Verification items for the finished model (mm, model axes). A direction names the side the tool comes from. Give positions to 0.01 mm unless a question says otherwise; leave off trailing zeros. Use a Markdown table: item, result.
from build123d import *

# Parameters (mm, degrees)
SKETCH1_W                = 94
SKETCH1_H                = 130
BOSS_EXTRUDE1_DEPTH      = 9.5
SKETCH2_W                = 90.5
SKETCH2_H                = 126.5
CUT_EXTRUDE1_DEPTH       = 2.5
SKETCH3_W                = 70
SKETCH3_H                = 24
CUT_EXTRUDE2_DEPTH       = 8
SKETCH4_W                = 70
SKETCH4_H                = 77
CUT_EXTRUDE3_DEPTH       = 2
SKETCH5_W                = 23
SKETCH5_H                = 3.5
CUT_EXTRUDE4_DEPTH       = 8.5
SKETCH6_W                = 6
SKETCH6_H                = 18
CUT_EXTRUDE5_DEPTH       = 3.5
SKETCH7_W                = 43
SKETCH7_H                = 7.5
CUT_EXTRUDE6_DEPTH       = 3
FILLET1_R                = 2
SKETCH9_R                = 2.75
CUT_EXTRUDE7_DEPTH       = 5
SKETCH12_W               = 6.2
SKETCH12_H               = 6.2
CUT_EXTRUDE9_DEPTH       = 3
SKETCH13_W               = 3.2
SKETCH13_H               = 6.2
CUT_EXTRUDE10_DEPTH      = 6
CUT_EXTRUDE10_DEPTH_BACK = 5.5
FILLET2_R                = 1
SKETCH14_R               = 4
BOSS_EXTRUDE2_DEPTH      = 3
SKETCH15_R               = 2.8
CUT_EXTRUDE11_DEPTH      = 1.5
SKETCH16_R               = 2.4
CUT_EXTRUDE12_DEPTH      = 1.5
SKETCH18_W               = 4
SKETCH18_H               = 6
SKETCH18_W_2             = 2
SKETCH18_H_2             = 4
SKETCH18_H_3             = 1
BOSS_EXTRUDE3_DEPTH      = 1


with BuildPart() as part:
    # Sketch1 → Boss-Extrude1 (new body)
    with BuildSketch(Plane(origin=(0, 7, 0), x_dir=(1, 0, 0), z_dir=(0, 1, 0))):
        with Locations((47, 65)):
            Rectangle(SKETCH1_W, SKETCH1_H)
    extrude(amount=-BOSS_EXTRUDE1_DEPTH)

    # Sketch2 → Cut-Extrude1 (cut)
    with BuildSketch(Plane.XZ.offset(2.5)):
        with Locations((47, -65)):
            Rectangle(SKETCH2_W, SKETCH2_H)
    extrude(amount=-CUT_EXTRUDE1_DEPTH, mode=Mode.SUBTRACT)

    # Sketch3 → Cut-Extrude2 (cut, through all)
    with BuildSketch(Plane.XZ):
        with Locations((47, -100)):
            Rectangle(SKETCH3_W, SKETCH3_H)
    extrude(amount=-CUT_EXTRUDE2_DEPTH, mode=Mode.SUBTRACT)

    # Sketch4 → Cut-Extrude3 (cut)
    with BuildSketch(Plane(origin=(0, 7, 0), x_dir=(-1, 0, 0), z_dir=(0, 1, 0))):
        with Locations((-47, -44.5)):
            Rectangle(SKETCH4_W, SKETCH4_H)
    extrude(amount=-CUT_EXTRUDE3_DEPTH, mode=Mode.SUBTRACT)

    # Sketch5 → Cut-Extrude4 (cut, through all)
    with BuildSketch(Plane(origin=(0, 5, 0), x_dir=(-1, 0, 0), z_dir=(0, 1, 0))):
        with Locations((-39, -9.25)):
            Rectangle(SKETCH5_W, SKETCH5_H)
    extrude(amount=-CUT_EXTRUDE4_DEPTH, mode=Mode.SUBTRACT)

    # Sketch6 → Cut-Extrude5 (cut)
    with BuildSketch(Plane.XZ):
        with Locations((85, -100)):
            Rectangle(SKETCH6_W, SKETCH6_H)
    extrude(amount=-CUT_EXTRUDE5_DEPTH, mode=Mode.SUBTRACT)

    # Sketch7 → Cut-Extrude6 (cut)
    with BuildSketch(Plane.XZ):
        with Locations((33.5, -115.75)):
            Rectangle(SKETCH7_W, SKETCH7_H)
    extrude(amount=-CUT_EXTRUDE6_DEPTH, mode=Mode.SUBTRACT)

    # Fillet1
    fillet1_edges = [part.edges().sort_by_distance(p)[0] for p in [
        (94, 7, -65),
        (47, 7, 0),
        (0, 7, -65),
        (47, 7, -130),
        (94, 2.25, -130),
        (94, 2.25, 0),
        (0, 2.25, 0),
        (0, 2.25, -130),
    ]]
    fillet(fillet1_edges, radius=FILLET1_R)

    # Sketch9 → Cut-Extrude7 (cut)
    with BuildSketch(Plane(origin=(0, 5, 0), x_dir=(1, 0, 0), z_dir=(0, 1, 0))):
        with Locations((74, 58)):
            Circle(SKETCH9_R)
    extrude(amount=-CUT_EXTRUDE7_DEPTH, mode=Mode.SUBTRACT)

    # Sketch12 → Cut-Extrude9 (cut)
    with BuildSketch(Plane(origin=(0, 5, 0), x_dir=(1, 0, 0), z_dir=(0, 1, 0))):
        with Locations((74, 31)):
            Rectangle(SKETCH12_W, SKETCH12_H)
    extrude(amount=-CUT_EXTRUDE9_DEPTH, mode=Mode.SUBTRACT)

    # Sketch13 → Cut-Extrude10 (cut, two sides)
    with BuildSketch(Plane(origin=(0, 2, 0), x_dir=(1, 0, 0), z_dir=(0, 1, 0))) as cut_extrude10_sk:
        with Locations((74, 31)):
            Rectangle(SKETCH13_W, SKETCH13_H)
    extrude(amount=CUT_EXTRUDE10_DEPTH, mode=Mode.SUBTRACT)
    extrude(cut_extrude10_sk.sketch, amount=-CUT_EXTRUDE10_DEPTH_BACK, mode=Mode.SUBTRACT)

    # Fillet2
    fillet2_edges = [part.edges().sort_by_distance(p)[0] for p in [
        (77.1, 3.5, -34.1),
        (77.1, 3.5, -27.9),
        (70.9, 3.5, -27.9),
        (70.9, 3.5, -34.1),
    ]]
    fillet(fillet2_edges, radius=FILLET2_R)

    # Sketch14 → Boss-Extrude2 (add)
    with BuildSketch(Plane.XZ):
        with Locations((74, -58)):
            Circle(SKETCH14_R)
    extrude(amount=BOSS_EXTRUDE2_DEPTH)

    # Sketch15 → Cut-Extrude11 (cut)
    with BuildSketch(Plane(origin=(0, 0, 0), x_dir=(1, 0, 0), z_dir=(0, 1, 0))):
        with Locations((74, 58)):
            Circle(SKETCH15_R)
    extrude(amount=-CUT_EXTRUDE11_DEPTH, mode=Mode.SUBTRACT)

    # Sketch16 → Cut-Extrude12 (cut)
    with BuildSketch(Plane(origin=(0, -1.5, 0), x_dir=(1, 0, 0), z_dir=(0, 1, 0))):
        with Locations((74, 58)):
            Circle(SKETCH16_R)
    extrude(amount=-CUT_EXTRUDE12_DEPTH, mode=Mode.SUBTRACT)

    # Sketch18 → Boss-Extrude3 (add)
    with BuildSketch(Plane(origin=(0, 7, 0), x_dir=(1, 0, 0), z_dir=(0, 1, 0))):
        Polygon((17, 122), (17, 118), (19, 118), (19.993343468, 118), (19.993343468, 117), (15.993343468, 117), (15.993343468, 123), (19.993343468, 123), (19.993343468, 122), (19, 122), align=None)
        Polygon((66.993343468, 122), (63.993343468, 122), (63.993343468, 120.5), (66.993343468, 120.5), (66.993343468, 117), (62.993343468, 117), (62.993343468, 118), (65.993343468, 118), (65.993343468, 119.5), (62.993343468, 119.5), (62.993343468, 123), (66.993343468, 123), align=None)
        with Locations((23.493343468, 120)):
            Rectangle(SKETCH18_W, SKETCH18_H)
        with Locations((23.493343468, 120)):
            Rectangle(SKETCH18_W_2, SKETCH18_H_2, mode=Mode.SUBTRACT)
        Polygon((27.993343468, 122), (27.993343468, 118), (29.109404955, 118), (30.993343468, 118), (30.993343468, 117), (26.993343468, 117), (26.993343468, 123), (27.993343468, 123), align=None)
        with Locations((34.493343468, 120)):
            Rectangle(SKETCH18_W, SKETCH18_H)
        with Locations((34.493343468, 120)):
            Rectangle(SKETCH18_W_2, SKETCH18_H_2, mode=Mode.SUBTRACT)
        Polygon((49.493343468, 122), (50.493343468, 122), (50.493343468, 123), (46.493343468, 123), (46.493343468, 119.5), (47.493343468, 119.5), (49.493343468, 119.5), (49.493343468, 118), (47.956084084, 118), (46.493343468, 118), (46.493343468, 117), (50.493343468, 117), (50.493343468, 120.5), (49.493343468, 120.5), (47.493343468, 120.5), (47.493343468, 122), align=None)
        Polygon((37.993343468, 123), (41.993343468, 123), (41.993343468, 120), (40.353343468, 120), (41.993343468, 118.2), (41.993343468, 117), (40.993343468, 117), (40.993343468, 117.812757926), (39.000522912, 120), (38.993343468, 120), (38.993343468, 118.442496016), (38.993343468, 117), (37.993343468, 117), align=None)
        with Locations((39.993343468, 121.5)):
            Rectangle(SKETCH18_W_2, SKETCH18_H_3, mode=Mode.SUBTRACT)
        Polygon((55.993343468, 122), (52.993343468, 122), (52.993343468, 120.5), (55.993343468, 120.5), (55.993343468, 119.5), (52.993343468, 119.5), (52.993343468, 118), (55.993343468, 118), (55.993343468, 117), (51.993343468, 117), (51.993343468, 123), (55.993343468, 123), align=None)
        Polygon((58.493343468, 123), (60.493343468, 119.163331999), (60.493343468, 123), (61.493343468, 123), (61.493343468, 117), (60.493343468, 117), (58.493343468, 120.836668001), (58.493343468, 117), (57.493343468, 117), (57.493343468, 123), align=None)
        with Locations((70.493343468, 120)):
            Rectangle(SKETCH18_W, SKETCH18_H)
        with Locations((70.493343468, 120)):
            Rectangle(SKETCH18_W_2, SKETCH18_H_2, mode=Mode.SUBTRACT)
        Polygon((74.993343468, 117), (74.993343468, 120), (75.000522912, 120), (76.993343468, 117.812757926), (76.993343468, 117), (77.993343468, 117), (77.993343468, 118.2), (76.353343468, 120), (77.993343468, 120), (77.993343468, 123), (73.993343468, 123), (73.993343468, 117), align=None)
        with Locations((75.993343468, 121.5)):
            Rectangle(SKETCH18_W_2, SKETCH18_H_3, mode=Mode.SUBTRACT)
    extrude(amount=BOSS_EXTRUDE3_DEPTH)


solid = part.part
(1) Draft check along Z on faces 1 (the flat face through (47, 5, -44)), 2 (the flat face through (40, 8, -120.7)). Enter one of: +Z half, -Z half, draft (parallel to the pull), parting line (faces both ways), or undercut.
Results below:
| item | result |
|---|---|
| face 1 | undercut |
| face 2 | draft |
(2) Gauge pin test, flat ends, axial feed: P1, Ø6.5, axis at x = 85, z = -101, coming from the -Y side; P2, Ø5, axis at x = 17.5, z = -22, coming from the +Y side; P3, Ø0.5, axis at x = 48.5, y = 7.5, coming from the +Z side. Record the tip position at first contact, or that the pin passes through.
Results below:
| item | result |
|---|---|
| P1 | y = 0 |
| P2 | y = 5 |
| P3 | z = -117 |
(3) Material ranges on line 1 (Z direction, x = 74, y = -1.9); line 2 (Z direction, x = 74, y = 1.05); line 3 (X direction, y = 2.85, z = -58), recorded low to high.
Results below:
| item | result |
|---|---|
| line 1 | -130 to -128.25, -62 to -60.4, -55.6 to -54, -1.75 to 0 |
| line 2 | -130 to -112, -88 to -60.75, -55.25 to -34.1, -27.9 to 0 |
| line 3 | 0 to 71.25, 76.75 to 94 |
(4) Set-up check for faces 3 (the flat face through (0, 1, -64)), 4 (the flat face through (88, 2, -100)), 5 (the flat face through (54, 4, -112)): record each of +Z, -Z, +X, -X, +Y, -Y from which the full face is reachable in a straight line by a thin tool's end or side.
Results below:
| item | result |
|---|---|
| face 3 | +Z, -Z, -X, +Y, -Y |
| face 4 | -Y |
| face 5 | +Y, -Y |
